Build history of the part. All positions in model axes, mm. A direction names the side the tool comes from. Coordinates: 2 decimals unless noted, no trailing zeros. Order: outer loops, then holes, each group sorted by start corner. A loop starts at its lowest first (then second) coordinate and runs counter-clockwise, first axis right, second up. Notation, with made-up numbers: (28, 53) - (81, 53) arc R25 ccw to (81, 84) - close; hole circle Ø11 at (-36.5, 37). An arc over 180 degrees is marked (long way). One line per item, written item: value.
from build123d import *

# Parameters (mm, degrees)
F0_R     = 12.4968
F2_DEPTH = 42.9006
F1_W     = 17.4498
F1_H     = 17.4498
F3_DEPTH = 7.8994
F4_R     = 4.953
F5_DEPTH = 76.2


with BuildPart() as f2:
    # F0 (on Front) → F2 (new body)
    with BuildSketch(Plane.XZ):
        Circle(F0_R)
    extrude(amount=-F2_DEPTH)

    # F1 (on face) → F3 (join)
    with BuildSketch(Plane.XZ):
        Rectangle(F1_W, F1_H)
    extrude(amount=F3_DEPTH)

    # F4 (on face) → F5 (cut)
    with BuildSketch(Plane(origin=(0, 42.9006, 0), x_dir=(-1, 0, 0), z_dir=(0, 1, 0))):
        Circle(F4_R)
    extrude(amount=-F5_DEPTH, mode=Mode.SUBTRACT)


solid = f2.part
1. Band-saw the part on D-D, the plane z = 5.75. Give the cut face in (x, y), and give its area (3 significant figures).
Values found:
outline: (-11.1, 0) - (-8.72, 0) - (-8.72, -7.9) - (8.72, -7.9) - (8.72, 0) - (11.1, 0) - (11.1, 42.9) - (-11.1, 42.9) - close
area: 1,090 mm2
2. Band-saw the part on B-B, the plane x = 0. Give the cut face in (y, z), and give its area (3 significant figures).
Values found:
outline: (-7.9, -8.72) - (0, -8.72) - (0, -12.5) - (42.9, -12.5) - (42.9, -4.95) - (-7.9, -4.95) - close; (-7.9, 4.95) - (42.9, 4.95) - (42.9, 12.5) - (0, 12.5) - (0, 8.72) - (-7.9, 8.72) - close
area: 707 mm2
3. Flat gauge pins, fed straight in: P1, Ø12.5, axis at x = 2, z = -3, coming from the -Y side; P2, Ø9, axis at x = 0, z = 0, coming from the -Y side; P3, Ø8, axis at y = 36, z = 5, coming from the +X side; P4, Ø2.5, axis at y = -6, z = 0.5, coming from the -X side. Where does each tip first touch, or does it go through?
Values found:
P1: stops at y = -7.9
P2: passes through
P3: stops at x = 12.46
P4: stops at x = -8.72
4. Two-plate mould, pull along X, no slides. Class faces 1 (the face through (8.725, -4, 0)), 2 (the face through (11.92, 21.15, 3.75)), 3 (the face through (0.64, 17.86, 4.91)), 4 (the face through (0, -4, 8.725)): pulls with the +X half, pulls with the -X half, needs draft (parallel to the pull), parting line crosses it, or undercut.
Values found:
face 1: pulls with the +X half
face 2: parting line crosses it
face 3: undercut
face 4: needs draft
5. Probe line 1 along Z through (x, y) = (0, 31); line 2 along X through (y, z) = (18, -1.5); line 3 along Y through (x, z) = (4.5, -10.5). List the from-to ranges inside material, lowest first.
Values found:
line 1: z = -12.5 to -4.95, 4.95 to 12.5
line 2: x = -12.41 to -4.72, 4.72 to 12.41
line 3: y = 0 to 42.9
6. 3-axis set-ups, long thin cutter, end or side, ignore diameter. For faces 5 (the face through (0, -4, -8.725)), 6 (the face through (-0.2, 42.901, -5.4)), 7 (the face through (-8.725, -4, 0)): which of +Z, -Z, +X, -X, +Y, -Y reach the whole face in a straight line?
Values found:
face 5: -Z, +X, -X, -Y
face 6: +Z, -Z, +X, -X, +Y
face 7: +Z, -Z, -X, -Y
7. Band-saw the part on C-C, the plane y = 25.5. Give the cut face in (x, z).
Values found:
outline: circle Ø24.99 at (0, 0); hole circle Ø9.91 at (0, 0)
8. Band-saw the part on A-A, the plane z = 0. Give the cut face in (x, y), and give its area (3 significant figures).
Values found:
outline: (-12.5, 0) - (-8.72, 0) - (-8.72, -7.9) - (-4.95, -7.9) - (-4.95, 42.9) - (-12.5, 42.9) - close; (4.95, -7.9) - (8.72, -7.9) - (8.72, 0) - (12.5, 0) - (12.5, 42.9) - (4.95, 42.9) - close
area: 707 mm2
